Design review of the part built by this model. Coordinates are the model's own, in mm. Face numbers are marked on the shaded views. A direction names the side the tool comes from. Give positions to 0.01 mm unless a question says otherwise; leave off trailing zeros. Loops run counter-clockwise (first coordinate to the right, second up) from the corner with the lowest first, then second, coordinate; pieces in that order, holes last. Notation, with made-up numbers: (15, -15) -> (22, -15) arc R32 ccw to (22, 13) -> close; hole circle Ø8 at (-1, 27.25). An arc over 180 degrees is marked (long way). Answer in a Markdown table with one row per item. Add a question column.
(1) Consider section B-B on x = -9.5. Write out the cut boundary in (y, z).
(2) For line 1 (Z direction, x = -9.5, y = 6.55); line 2 (Z direction, x = -9.5, y = 5.7); line 3 (Y direction, x = -11.25, z = -4.25), list the stretches that pass through material, from the lowest coordinate up.
(3) Consider section C-C on y = 3. Write out the cut boundary in (x, z).
(4) For the marked faces 1, 2, 3 and 4, list the 3-axis set-ups (+Z, -Z, +X, -X, +Y, -Y) from which the entire face can be reached by the end or side of a thin tool; tool diameter is ignored.
(5) Draft analysis for pull direction Z (two halves, no side actions). For the marked faces 5, 6 and 7, state which applies: +Z half, -Z half, draft (parallel to the pull), parting line (faces both ways), or undercut.
(6) Consider section D-D on z = -1.25. Write out the cut boundary in (x, y), then the cut area to 3 significant figures.
(7) Consider section A-A on z = -9.5. Write out the cut boundary in (x, y), then the cut area to 3 significant figures.
(8) For pin 1 (3 mm diameter, centred on y = 0.5, z = -4, fed in from -X); pin 2 (2 mm diameter, centred on y = -2, z = 4, fed in from -X); pin 3 (2 mm diameter, centred on x = 3.5, y = 1, fed in from -Z), all flat-tipped, find the tip position at first contact; note any pin that passes through.
Autodesk Inventor part; units mm, degrees
ref_plane "YZ Plane" through (0, 0, 0) normal (1, 0, 0) x (0, 1, 0)
ref_plane "XZ Plane" through (0, 0, 0) normal (0, 1, 0) x (-1, 0, 0)
ref_plane "XY Plane" through (0, 0, 0) normal (0, 0, 1) x (1, 0, 0)
sketch "Boceto1" plane through (0, 0, 0) normal (0, 1, 0) x (-1, 0, 0)
  line L0 (5.4875, 5.487) -> (5.4875, 2.7435)
  line L1 (-5.487, 5.487) -> (-2.743, 5.487)
  line L2 (5.4875, 5.487) -> (2.744, 5.487)
  line L3 (-5.487, -5.487) -> (-5.487, -2.7435)
  line L4 (8.2308, 0.0003) -> (5.4875, 2.7435)
  line L5 (8.2308, 0.0003) -> (5.487, -2.7435)
  line L6 (0, -8.2305) -> (-2.7435, -5.487)
  line L7 (-8.2305, 0) -> (-5.487, -2.7435)
  line L8 (-5.487, 2.7435) -> (-8.2305, 0)
  line L9 (-2.743, 5.487) -> (0.0005, 8.2305)
  line L10 (0.0005, 8.2305) -> (2.744, 5.487)
  line L11 (2.7435, -5.487) -> (0, -8.2305)
  line L12 (5.487, -5.487) -> (2.7435, -5.487)
  line L13 (-2.7435, -5.487) -> (-5.487, -5.487)
  line L14 (5.4875, 5.487) -> (5.4875, 2.7435)
  line L15 (5.487, -2.7435) -> (5.487, -5.487)
  line L16 (-5.487, 5.487) -> (-2.743, 5.487)
  line L17 (2.744, 5.487) -> (5.4875, 5.487)
  line L18 (-5.487, -5.487) -> (-5.487, -2.7435)
  line L19 (-5.487, 2.7435) -> (-5.487, 5.487)
  arc A0 (1.8459, -2.0921) -> (0, -2.79) centre (0, 0) ccw
  line L20 (0, -2.79) -> (1.8459, -2.0921)
  dimension "d11" = 2.744
extrude "Extrusión1" add sketch "Boceto1" along normal mid plane 9 contours L0 L4 L5 L15 L12 L11 L6 L13 L3 L7 L8 L19 L1 L9 L10 L2 | L20 A0
sketch "Boceto2" plane through (0, 4.5, 0) normal (0, 1, 0) x (1, 0, 0)
  line L0 (0, -14) -> (-14, -14)
  line L1 (-14, -14) -> (-14, 0)
  line L2 (0, 14) -> (-14, 14)
  line L3 (-14, 14) -> (-14, 0)
  line L4 (0, -14) -> (14, -14)
  line L5 (14, -14) -> (14, 0)
  line L6 (0, 14) -> (14, 14)
  line L7 (14, 14) -> (14, 0)
  line L8 (-14, -14) -> (-14, -9.5)
  circle A0 centre (-9.5, -9.5) radius 1.5
  circle A1 centre (9.5, -9.5) radius 1.5
  circle A2 centre (9.5, 9.5) radius 1.5
  circle A3 centre (-9.5, 9.5) radius 1.5
  point P0 (0, 0)
  dimension "d26" = 4.5
  dimension "d28" = 3
  dimension "d31" = 360
extrude "Extrusión2" add sketch "Boceto2" along normal blind 3 contours L0 L1 L3 L2 L6 L7 L5 L4 | A0 | A1 | A2 | A3
sketch "Boceto5" plane through (0, -4.5, 0) normal (0, -1, 0) x (1, 0, 0)
  arc A0 (0, -3) -> (-1.9849, -2.2495) centre (0, 0) ccw
  line L0 (0, -3) -> (-1.9849, -2.2495)
  dimension "d48" = 6
extrude "Extrusión5" cut sketch "Boceto5" along normal mid plane 100
fillet "Empalme1" radius 2 4 edges at (-14, 4.5, 0) (0, 4.5, -14) (14, 4.5, 0) (0, 4.5, 14)
sketch "Boceto7" plane through (0, 4.5, 0) normal (0, -1, 0) x (1, 0, 0)
  circle A0 centre (-9.5, 9.5) radius 1.5
  circle A1 centre (-9.5, -9.5) radius 1.5
  circle A2 centre (9.5, -9.5) radius 1.5
  circle A3 centre (9.5, 9.5) radius 1.5
  point P0 (0, 0)
  dimension "d75" = 3
  dimension "d78" = 360
extrude "Extrusión7" cut sketch "Boceto7" against normal mid plane 190
properties part number "Acople Motor 1"
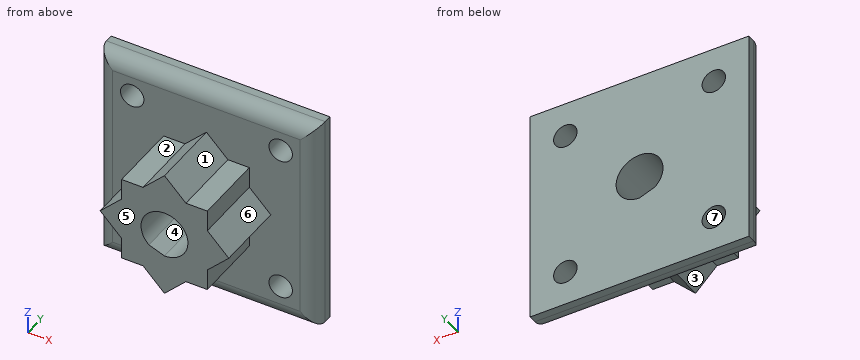
Values follow:
| question | item | result |
|---|---|---|
| 1 | outline | (4.5, -12) arc R2 ccw to (6.5, -14) -> (7.5, -14) -> (7.5, -11) -> (4.5, -11) -> close; (4.5, -8) -> (7.5, -8) -> (7.5, 8) -> (4.5, 8) -> close; (4.5, 11) -> (7.5, 11) -> (7.5, 14) -> (6.5, 14) arc R2 ccw to (4.5, 12) -> close |
| 2 | line 1 | -14 to -11, -8 to 8, 11 to 14 |
| 2 | line 2 | -13.83 to -11, -8 to 8, 11 to 13.83 |
| 2 | line 3 | 4.5 to 7.5 |
| 3 | outline | (-8.23, 0) -> (-5.49, -2.74) -> (-5.49, -5.49) -> (-2.74, -5.49) -> (0, -8.23) -> (2.74, -5.49) -> (5.49, -5.49) -> (5.49, -2.74) -> (8.23, 0) -> (5.49, 2.74) -> (5.49, 5.49) -> (2.74, 5.49) -> (0, 8.23) -> (-2.74, 5.49) -> (-5.49, 5.49) -> (-5.49, 2.74) -> close; hole (-1.98, -2.25) -> (0, -3) arc R3 ccw (long way) to start |
| 4 | face 1 | +Z, +X, -Y |
| 4 | face 2 | +Z, -X, -Y |
| 4 | face 3 | -Z, -X, -Y |
| 4 | face 4 | +Y, -Y |
| 5 | face 5 | draft |
| 5 | face 6 | +Z half |
| 5 | face 7 | undercut |
| 6 | outline | (-14, 6.5) arc R2 ccw to (-12, 4.5) -> (-6.98, 4.5) -> (-6.98, -4.5) -> (-2.73, -4.5) -> (-2.73, 7.5) -> (-14, 7.5) -> close; (2.73, -4.5) -> (6.98, -4.5) -> (6.98, 4.5) -> (12, 4.5) arc R2 ccw to (14, 6.5) -> (14, 7.5) -> (2.73, 7.5) -> close |
| 6 | area | 142 mm2 |
| 7 | outline | (-14, 6.5) arc R2 ccw to (-12, 4.5) -> (-11, 4.5) -> (-11, 7.5) -> (-14, 7.5) -> close; (-8, 4.5) -> (8, 4.5) -> (8, 7.5) -> (-8, 7.5) -> close; (11, 4.5) -> (12, 4.5) arc R2 ccw to (14, 6.5) -> (14, 7.5) -> (11, 7.5) -> close |
| 7 | area | 64.3 mm2 |
| 8 | pin 1 | x = -5.73 |
| 8 | pin 2 | x = -5.49 |
| 8 | pin 3 | z = -5.73 |
